Autodesk Inventor part; units mm, degrees
ref_plane "YZ Plane" through (0, 0, 0) normal (1, 0, 0) x (0, 1, 0)
ref_plane "XZ Plane" through (0, 0, 0) normal (0, 1, 0) x (-1, 0, 0)
ref_plane "XY Plane" through (0, 0, 0) normal (0, 0, 1) x (1, 0, 0)
sketch "Sketch1" plane through (0, 0, 0) normal (0, 0, 1) x (1, 0, 0)
  line L0 (0, 0) -> (0, 50.8)
  line L1 (0, 50.8) -> (3.175, 50.8)
  line L2 (3.175, 50.8) -> (3.175, 3.175)
  line L3 (3.175, 3.175) -> (50.8, 3.175)
  line L4 (0, 0) -> (50.8, 0)
  line L5 (50.8, 3.175) -> (50.8, 0)
  dimension "d0" = 50.8
  dimension "d1" = 3.175
  dimension "d2" = 47.625
  dimension "d5" = 50.8
  dimension "d6" = 3.175
extrude "Extrusion1" add sketch "Sketch1" along normal blind 25.4
sketch "Sketch2" plane through (3.175, 3.175, 0) normal (1, 0, 0) x (0, 0, -1)
  line L0 (0, 47.625) -> (-25.4, 47.625)
  line L1 (-25.4, 0) -> (-25.4, 47.625)
  line L2 (0, 0) -> (-25.4, 0)
  point P0 (0, -3.175)
  point P1 (-12.7, 34.925)
  point P2 (-12.7, 9.525)
  dimension "d16" = 12.7
  dimension "d17" = 12.7
  dimension "d19" = 12.7
  dimension "d34" = 25.4
hole "Hole1" at (3.175, 38.1, 12.7) at (3.175, 12.7, 12.7) direction (-1, 0, 0) diameter 5.08 end through all
sketch "Sketch3" plane through (3.175, 3.175, 0) normal (0, 1, 0) x (1, 0, 0)
  line L0 (47.625, -25.4) -> (0, -25.4)
  line L1 (0, 0) -> (0, -25.4)
  line L2 (47.625, 0) -> (47.625, -25.4)
  point P0 (-3.175, 0)
  point P1 (9.525, -12.7)
  point P2 (34.925, -12.7)
  dimension "d23" = 12.7
  dimension "d25" = 12.7
  dimension "d26" = 12.7
  dimension "d35" = 25.4
hole "Hole2" at (12.7, 3.175, 12.7) at (38.1, 3.175, 12.7) direction (0, -1, 0) diameter 5.08 end through all
equation "\"d2\" = d0 - d6"
equation "\"d6\" = d1"
properties part number "Centerpiece-90CornerBracket" material "Aluminum 6061-AHC"
Verification items for the finished model (mm, model axes). A direction names the side the tool comes from. Round coordinates to 2 decimals unless told otherwise and drop trailing zeros. Write each loop counter-clockwise with the first axis right and the second up, starting at its lowest first coordinate (ties: lowest second). Pieces come first, ordered by that corner, then holes. Notation, with made-up numbers: (47.25, 77.5) - (67.25, 77.5) arc R10 cw to (67.25, 86.5) - close; hole circle Ø2 at (76.5, 68). An arc over 180 degrees is marked (long way). Answer as a JSON object with one key per item and string values. Group by question number.
Q1. Thickness scan on line 1 (Y direction, x = 2, z = 12.7); line 2 (Z direction, x = 2, y = 38); line 3 (X direction, y = 6.5, z = 2.5) (3 decimals). Record the ranges inside material, lowest first.
Q2. Section check B-B, the plane x = 38.1. Enter the section's corners in (y, z) (3 decimals), plus the area to 3 significant figures.
Q3. Section check A-A, the plane z = 12.7. Enter the section's corners in (x, y) (3 decimals).
Q4. Mould release check, pull along Z, two halves, no side actions. Record for faces 3 (the cylindrical face through (40.58, 1.57, 12.15)), 4 (the flat face through (27, 3.175, 13)), 5 (the flat face through (3, 14, 25.4)), 6 (the cylindrical face through (1.57, 40.58, 13.25)): released by +Z, released by -Z, zero draft, split by the parting line, or undercut.
Q5. Tool access check on faces 1 (the flat face through (3.175, 27, 13)), 2 (the flat face through (50.8, 2, 13)). Record the directions out of +Z, -Z, +X, -X, +Y, -Y that give a thin tool (end or side, any length) a straight path to the whole face; none if there is none.
Q6. Go/stop test with flat-tipped pins: pin 1 Ø12.5 at (y, z) = (19, 8) entering from +X (3 decimals); pin 2 Ø4.5 at (x, z) = (38.1, 12.7) entering from +Y. Record where each tip stops, or that it passes through.
Q7. Section check D-D, the plane z = 23.75. Enter the section's corners in (x, y) (3 decimals).
Found:
{
 "1": {"line 1": "y = 0 to 10.16, 15.24 to 35.56, 40.64 to 50.8", "line 2": "z = 0 to 10.16, 15.24 to 25.4", "line 3": "x = 0 to 3.175"},
 "2": {"outline": "(0, 0) - (3.175, 0) - (3.175, 10.16) - (0, 10.16) - close; (0, 15.24) - (3.175, 15.24) - (3.175, 25.4) - (0, 25.4) - close", "area": "64.5 mm^2"},
 "3": {"outline": "(0, 0) - (10.16, 0) - (10.16, 3.175) - (3.175, 3.175) - (3.175, 10.16) - (0, 10.16) - close; (0, 15.24) - (3.175, 15.24) - (3.175, 35.56) - (0, 35.56) - close; (0, 40.64) - (3.175, 40.64) - (3.175, 50.8) - (0, 50.8) - close; (15.24, 0) - (35.56, 0) - (35.56, 3.175) - (15.24, 3.175) - close; (40.64, 0) - (50.8, 0) - (50.8, 3.175) - (40.64, 3.175) - close"},
 "4": {"face 3": "undercut", "face 4": "zero draft", "face 5": "released by +Z", "face 6": "undercut"},
 "5": {"face 1": "+Z, -Z, +X, +Y", "face 2": "+Z, -Z, +X, +Y, -Y"},
 "6": {"pin 1": "stops at x = 3.175", "pin 2": "passes through"},
 "7": {"outline": "(0, 0) - (50.8, 0) - (50.8, 3.175) - (3.175, 3.175) - (3.175, 50.8) - (0, 50.8) - close"}
}
